Job drawing, mm, ordinate dimensions from the low corner. One solid piece. A direction names the side the tool comes from. Give positions to 0.01 mm unless a question says otherwise; leave off trailing zeros. Order: outer loops, then holes, each group sorted by start corner. A loop starts at its lowest first (then second) coordinate and runs counter-clockwise, first axis right, second up. Notation, with made-up numbers: (58.5, -2.5) - (116.5, -2.5) arc R26 ccw to (116.5, 21.5) - close; hole circle Ø5 at (49, 88.5). An arc over 180 degrees is marked (long way). Write each question's results on one line, items separated by ' | '. Start each with the question number.
1) Tool access for the marked faces 1, 2 and 3: list every direction of +Z, -Z, +X, -X, +Y, -Y with a clear straight run to the whole face (end or side of a thin tool).
2) Drill centre lines: line 1 along X through (y, z) = (29, 19) (1 decimal); line 2 along X through (y, z) = (25.5, 17) (1 decimal); line 3 along Y through (x, z) = (21, 29.5). Where is each one in solid material? Low to high. Write a range as from..to.
3) Cut at A-A on y = 10.16. List the corners of the cut face in (x, z).
4) Cut at C-C on y = 4. List the corners of the cut face in (x, z), plus the area to 3 significant figures.
5) Drop flat-ended pins along their axis: pin 1 Ø3 at (y, z) = (9.5, 9) entering from -X; pin 2 Ø12 at (x, z) = (48.5, 20.5) entering from -Y; pin 3 Ø10 at (y, z) = (22, 11) entering from +X; pin 4 Ø5 at (x, y) = (28.5, 22.5) entering from +Z. Give the stop position or say it passes through.
6) Cut at B-B on z = 19.05. State how many separate pieces and enclosed holes the cut face has, plus the area to 3 significant figures.
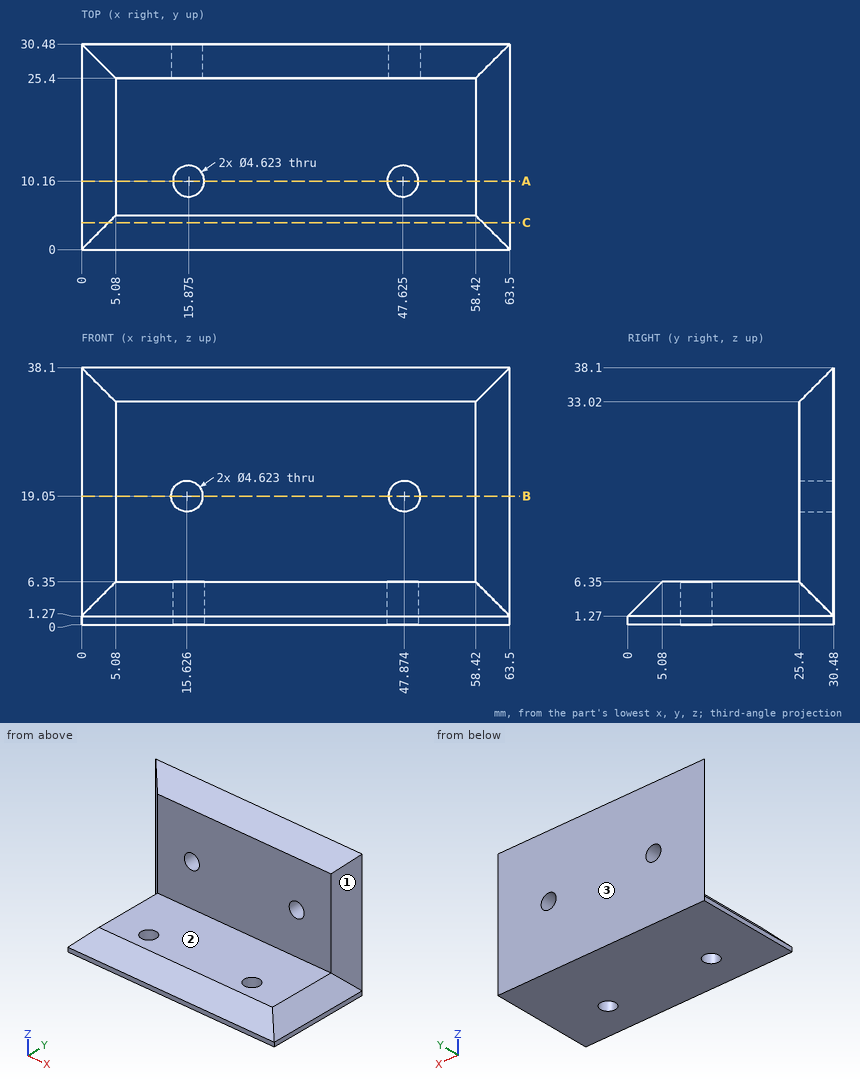
Results:
1) face 1: +Z, +X, -Y | face 2: +Z, +X, -X, -Y | face 3: +Z, -Z, +X, -X, +Y
2) line 1: 1.5..13.3, 17.9..45.6, 50.2..62 | line 2: 5..14.6, 16.7..46.8, 48.9..58.5 | line 3: 25.4..30.48
3) outline: (0, 0) - (13.56, 0) - (13.56, 6.35) - (5.08, 6.35) - (0, 1.27) - close; (18.19, 0) - (45.31, 0) - (45.31, 6.35) - (18.19, 6.35) - close; (49.94, 0) - (63.5, 0) - (63.5, 1.27) - (58.42, 6.35) - (49.94, 6.35) - close
4) outline: (0, 0) - (63.5, 0) - (63.5, 1.27) - (59.5, 5.27) - (4, 5.27) - (0, 1.27) - close | area: 319 mm^2
5) pin 1: through | pin 2: y = 25.4 | pin 3: x = 60.02 | pin 4: z = 6.35
6) separate pieces: 3 | enclosed holes: 0 | area: 250 mm^2
